Geometry check sheet. Reference: the model listing, model coordinates, mm. A direction names the side the tool comes from. Round coordinates to 2 decimals unless told otherwise and drop trailing zeros. Order: outer loops, then holes, each group sorted by start corner. A loop starts at its lowest first (then second) coordinate and runs counter-clockwise, first axis right, second up. Notation, with made-up numbers: (-7, 30.5) - (31, 30.5) arc R27 cw to (31, 62.5) - close; hole circle Ø9 at (80.5, 79.5). An arc over 180 degrees is marked (long way). Use a Markdown table: item, result. Add a question column.
(1) Thickness scan on line 1 along X through (y, z) = (46, 0); line 2 along Z through (x, y) = (5, 81.5); line 3 along X through (y, z) = (14, -3.5). Record the ranges inside material, lowest first. Write a range as [from, to].
(2) Gauge pin test, flat ends, axial feed: P1, Ø3, axis at x = -5.5, z = -10.5, coming from the +Y side; P2, Ø1.5, axis at x = 12.5, y = 67.5, coming from the +Z side; P3, Ø12, axis at x = -19, y = 40.5, coming from the -Z side. Record the tip position at first contact, or that the pin passes through.
(3) Access from +Z, -Z, +X, -X, +Y, -Y to the whole of each face (thin tool, end or side, straight path). Record for faces 3 (the face through (-16.81, 3.7, 12.35)), 4 (the face through (-6.448, 3.698, -13.544)), 5 (the face through (20.76, 3.8, -3.27)).
(4) Mould release check, pull along Z, two halves, no side actions. Record for faces 1 (the face through (19.103, 3.698, 8.387)), 2 (the face through (1.32, 53, -29.97)): released by +Z, released by -Z, zero draft, split by the parting line, or undercut.
(5) Section check B-B on x = 0. Record the boundary of the cut face in (y, z).
(6) Section check D-D on y = 24. Record the boundary of the cut face in (x, z), then the cut area to 3 significant figures.
(7) Section check C-C on z = 19.5. Record the boundary of the cut face in (x, y).
(8) Section check A-A on z = 0. Record the boundary of the cut face in (x, y), then the cut area to 3 significant figures.
```python
from build123d import *

# Parameters (mm, degrees)
SKETCH1_R                            = 20
BOSS_EXTRUDE1_DEPTH                  = 10
SKETCH1_R_2                          = 40
SKETCH1_R_3                          = 36
BOSS_EXTRUDE1_2_DEPTH                = 10
BOSS_EXTRUDE2_REACH                  = 89.446
BOSS_EXTRUDE2_END_RADIUS             = 36
BOSS_EXTRUDE2_START                  = 30
BOSS_EXTRUDE2_DIRECTION_2_REACH      = 89.446
BOSS_EXTRUDE2_DIRECTION_2_END_RADIUS = 20
CIRPATTERN1_COUNT                    = 12
SKETCH5_R                            = 1.735695499
BOSS_EXTRUDE3_DEPTH                  = 5
SCALE1_SCALE                         = 0.75
SKETCH6_R                            = 30
SKETCH6_R_2                          = 27
BOSS_EXTRUDE4_DEPTH                  = 100
SKETCH7_R                            = 9.5
BOSS_EXTRUDE5_DEPTH                  = 100


with BuildPart() as part:
    # Sketch1 → Boss-Extrude1 (new body)
    with BuildSketch(Plane(origin=(0, 0, 0), x_dir=(1, 0, 0), z_dir=(0, 1, 0))):
        with Locations(Location((0, 0, 0), (0, 0, 270))):
            Circle(SKETCH1_R)
    extrude(amount=BOSS_EXTRUDE1_DEPTH)


with BuildPart() as body_2:
    # Sketch1 → Boss-Extrude1 2 (new body)
    with BuildSketch(Plane(origin=(0, 0, 0), x_dir=(1, 0, 0), z_dir=(0, 1, 0))):
        with Locations(Location((0, 0, 0), (0, 0, 270))):
            Circle(SKETCH1_R_2)
        with Locations(Location((0, 0, 0), (0, 0, 270))):
            Circle(SKETCH1_R_3, mode=Mode.SUBTRACT)
    extrude(amount=BOSS_EXTRUDE1_2_DEPTH)


    add(part.part)  # Boss-Extrude2 merges part
    # Boss-Extrude2: up to this cylinder (the profile starts inside it)
    boss_extrude2_end = Plane(origin=(0, 5, 0), z_dir=(0, -1, 0)) * Cylinder(BOSS_EXTRUDE2_END_RADIUS, 251.892, mode=Mode.PRIVATE)
    # Sketch4 → Boss-Extrude2 (add, up to the surface)
    with BuildSketch(Plane(origin=(0, 0, 0), x_dir=(0, 0, -1), z_dir=(1, 0, 0)).offset(BOSS_EXTRUDE2_START), mode=Mode.PRIVATE) as boss_extrude2_sk1:
        Polygon((2.097443169, 0), (4.031443844, 10), (5.315133993, 10), (3.381133319, 0), align=None)
    boss_extrude2_tool1 = extrude(boss_extrude2_sk1.sketch, amount=BOSS_EXTRUDE2_REACH, mode=Mode.PRIVATE) & boss_extrude2_end
    boss_extrude2 = boss_extrude2_tool1.solids().sort_by_distance((30, 5, -3.706289))[0]
    add(boss_extrude2)

    # Boss-Extrude2 direction 2: up to this cylinder (the profile starts outside it)
    boss_extrude2_direction_2_end = Plane(origin=(0, 5, 0), z_dir=(0, -1, 0)) * Cylinder(BOSS_EXTRUDE2_DIRECTION_2_END_RADIUS, 219.892, mode=Mode.PRIVATE)
    # Sketch4 → Boss-Extrude2 direction 2 (add, up to the surface)
    with BuildSketch(Plane(origin=(0, 0, 0), x_dir=(0, 0, -1), z_dir=(1, 0, 0)).offset(BOSS_EXTRUDE2_START), mode=Mode.PRIVATE) as boss_extrude2_direction_2_sk1:
        Polygon((2.097443169, 0), (4.031443844, 10), (5.315133993, 10), (3.381133319, 0), align=None)
    boss_extrude2_direction_2_tool1 = extrude(boss_extrude2_direction_2_sk1.sketch, amount=-BOSS_EXTRUDE2_DIRECTION_2_REACH, mode=Mode.PRIVATE) - boss_extrude2_direction_2_end
    boss_extrude2_direction_2 = boss_extrude2_direction_2_tool1.solids().sort_by_distance((30, 5, -3.706289))[0]
    add(boss_extrude2_direction_2)
    boss_extrude2 = boss_extrude2 + boss_extrude2_direction_2  # both directions under the feature's name, for the pattern or mirror that repeats it

    # CirPattern1: Boss-Extrude2 ×12 about axis
    cirpattern1_axis = Axis((0, 0, 0), (0, 1, 0))
    for i in range(1, CIRPATTERN1_COUNT):
        add(boss_extrude2.rotate(cirpattern1_axis, i * 360 / CIRPATTERN1_COUNT))

    # Sketch5 → Boss-Extrude3 (add)
    with BuildSketch(Plane(origin=(0, 10, 0), x_dir=(1, 0, 0), z_dir=(0, 1, 0))):
        with Locations(Location((-14.887021655, 0, 0), (0, 0, 270))):
            Circle(SKETCH5_R)
        with Locations(Location((-7.443510827, 12.89253894, 0), (0, 0, 270))):
            Circle(SKETCH5_R)
        with Locations(Location((7.443510827, 12.89253894, 0), (0, 0, 270))):
            Circle(SKETCH5_R)
        with Locations(Location((14.887021655, 0, 0), (0, 0, 270))):
            Circle(SKETCH5_R)
        with Locations(Location((7.443510827, -12.89253894, 0), (0, 0, 270))):
            Circle(SKETCH5_R)
        with Locations(Location((-7.443510827, -12.89253894, 0), (0, 0, 270))):
            Circle(SKETCH5_R)
    extrude(amount=BOSS_EXTRUDE3_DEPTH)


with BuildPart() as body_2_1:
    # Scale1: scaled about (0, 0, 0)
    add(body_2.part.scale(SCALE1_SCALE))

    # Sketch6 → Boss-Extrude4 (add)
    with BuildSketch(Plane(origin=(0, 7.5, 0), x_dir=(1, 0, 0), z_dir=(0, 1, 0))):
        with Locations(Location((0, 0, 0), (0, 0, 270))):
            Circle(SKETCH6_R)
        with Locations(Location((0, 0, 0), (0, 0, 93.340075949))):
            Circle(SKETCH6_R_2, mode=Mode.SUBTRACT)
    extrude(amount=BOSS_EXTRUDE4_DEPTH)

    # Sketch7 → Boss-Extrude5 (add)
    with BuildSketch(Plane(origin=(0, 7.5, 0), x_dir=(1, 0, 0), z_dir=(0, 1, 0))):
        with Locations(Location((0, 0, 0), (0, 0, 270))):
            Circle(SKETCH7_R)
    extrude(amount=BOSS_EXTRUDE5_DEPTH)


solid = body_2_1.part
```
Check sheet entries:
| question | item | result |
|---|---|---|
| 1 | line 1 | x = [-30, -27], [-9.5, 9.5], [27, 30] |
| 1 | line 2 | z = [-29.58, -26.53], [-8.08, 8.08], [26.53, 29.58] |
| 1 | line 3 | x = [-29.8, -26.77], [-8.83, 8.83], [26.77, 29.8] |
| 2 | P1 | stops at y = 11.25 |
| 2 | P2 | stops at z = 27.6 |
| 2 | P3 | stops at z = -27.04 |
| 3 | face 3 | +Y |
| 3 | face 4 | none |
| 3 | face 5 | -Y |
| 4 | face 1 | undercut |
| 4 | face 2 | split by the parting line |
| 5 | outline | (0, -30) - (107.5, -30) - (107.5, -27) - (0, -27) - close; (0, -15) - (7.5, -15) - (7.5, -9.5) - (107.5, -9.5) - (107.5, 9.5) - (7.5, 9.5) - (7.5, 15) - (0, 15) - close; (0, 27) - (107.5, 27) - (107.5, 30) - (0, 30) - close |
| 6 | outline | circle Ø60 at (0, 0); circle Ø19 at (0, 0); hole circle Ø54 at (0, 0) |
| 6 | area | 821 mm2 |
| 7 | outline | (-22.8, 0) - (-18.67, 0) - (-18.67, 107.5) - (-22.8, 107.5) - close; (-9.44, 0) - (-8.33, 0) - (-6.66, 7.5) - (-7.77, 7.5) - close; (1.57, 0) - (2.54, 0) - (3.99, 7.5) - (3.02, 7.5) - close; (13.07, 0) - (14.19, 0) - (15.86, 7.5) - (14.75, 7.5) - close; (18.67, 0) - (22.8, 0) - (22.8, 107.5) - (18.67, 107.5) - close |
| 8 | outline | (-30, 0) - (-27, 0) - (-27, 107.5) - (-30, 107.5) - close; (-15, 0) - (15, 0) - (15, 7.5) - (12.47, 7.5) - (12.47, 11.25) - (9.86, 11.25) - (9.86, 7.5) - (9.5, 7.5) - (9.5, 107.5) - (-9.5, 107.5) - (-9.5, 7.5) - (-9.86, 7.5) - (-9.86, 11.25) - (-12.47, 11.25) - (-12.47, 7.5) - (-15, 7.5) - close; (27, 0) - (30, 0) - (30, 107.5) - (27, 107.5) - close |
| 8 | area | 2,790 mm2 |
